Autodesk Inventor part; units mm, degrees
ref_plane "YZ Plane" through (0, 0, 0) normal (1, 0, 0) x (0, 1, 0)
ref_plane "XZ Plane" through (0, 0, 0) normal (0, 1, 0) x (-1, 0, 0)
ref_plane "XY Plane" through (0, 0, 0) normal (0, 0, 1) x (1, 0, 0)
sketch "スケッチ1" plane through (0, 0, 0) normal (0, 0, 1) x (1, 0, 0)
  circle A0 centre (0, 0) radius 1.5
  dimension "d0" = 3
extrude "押し出し1" add sketch "スケッチ1" along normal blind 4
sketch "スケッチ2" plane through (0, 0, 0) normal (0, 0, -1) x (-1, 0, 0)
  circle A0 centre (0, 0) radius 2.75
  dimension "d3" = 5.5
extrude "押し出し2" add sketch "スケッチ2" along normal blind 2
fillet "フィレット1" radius 2 1 edges at (2.75, 0, -2)
thread "ねじ1"
properties part number "ネジ鍋m3,04" material "鋼、高強度、低合金"
Part model, mm, in its own coordinate system. A direction names the side the tool comes from. Give positions to 0.01 mm unless a question says otherwise; leave off trailing zeros. Write each loop counter-clockwise with the first axis right and the second up, starting at its lowest first coordinate (ties: lowest second). Pieces come first, ordered by that corner, then holes.
1) Probe L1, parallel to Y at x = 1.3, z = 2.5; L2, parallel to Y at x = 0, z = 2. List the from-to ranges inside material, lowest first.
Resolved:
L1: y = -0.75 to 0.75
L2: y = -1.5 to 1.5
2) Pin check, flat tips, straight feed: pin 1 (1.5 mm diameter, centred on y = -2, z = 1.5, fed in from -X); pin 2 (1 mm diameter, centred on y = 1.5, z = 2.5, fed in from +X); pin 3 (2 mm diameter, centred on y = -1, z = 2, fed in from +X). Stop position of each tip, or through.
Resolved:
pin 1: stops at x = -0.83
pin 2: stops at x = 1.12
pin 3: stops at x = 1.5
3) Cut at A-A on z = 2.5. Write the cut outline in (x, y).
Resolved:
outline: circle Ø3 at (0, 0)
4) Which spindle directions (+Z, -Z, +X, -X, +Y, -Y) get a long thin tool onto all of the face, cutting with end or side? Do faces 1 (the face through (-1.5, -0.07, 1.97)), 2 (the face through (0, 0, -2)). Say none if no direction does.
Resolved:
face 1: +Z
face 2: -Z, +X, -X, +Y, -Y
